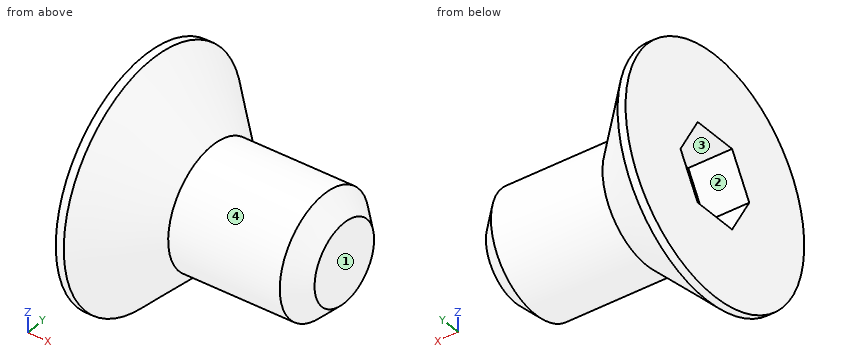
from build123d import *

# Parameters (mm, degrees)
CUT_EXTRUDE1_DEPTH = 1.1


with BuildPart() as part:
    # Sketch1 → Revolve1 (revolve)
    with BuildSketch(Plane.XY, mode=Mode.PRIVATE) as revolve1_sk:
        Polygon((0, -1.5), (2.8, -1.5), (3.3, -1), (3.3, 0), (-1.7, 0), (-1.7, -3), (-1.5, -3), align=None)
    revolve(revolve1_sk.sketch.rotate(Axis((-1.7, 0, 0), (1, 0, 0)), 270), axis=Axis((-1.7, 0, 0), (1, 0, 0)))

    # Sketch2 → Cut-Extrude1 (cut)
    with BuildSketch(Plane.ZY.offset(1.7)):
        Polygon((0, 1.154700538), (-1, 0.577350269), (-1, -0.577350269), (0, -1.154700538), (1, -0.577350269), (1, 0.577350269), align=None)
    extrude(amount=-CUT_EXTRUDE1_DEPTH, mode=Mode.SUBTRACT)


solid = part.part
Work out the finished part from the listing and answer in its coordinate system (mm). Face numbers are marked on the shaded views. Round coordinates to 2 decimals unless told otherwise and drop trailing zeros. Write each loop counter-clockwise with the first axis right and the second up, starting at its lowest first coordinate (ties: lowest second). Pieces come first, ordered by that corner, then holes.
1) The mould has two halves that part along Y. Classify the marked faces 1, 2, 3 and 4: pulls with the +Y half, pulls with the -Y half, needs draft (parallel to the pull), parting line crosses it, or undercut.
2) A cutting plane is placed at B-B (y = 0). Give the vertices of the cut face in (x, z).
3) A cutting plane is placed at A-A (x = -1.25). Give the vertices of the cut face in (y, z).
4) A cutting plane is placed at C-C (x = 0.1). Give the vertices of the cut face in (y, z), plus the area to 3 significant figures.
5) Given pin 1 Ø1.5 at (x, z) = (2.5, -1) entering from +Y; pin 2 Ø1.5 at (x, y) = (1, 1.5) entering from +Z; pin 3 Ø1 at (x, z) = (1, -1.5) entering from -Y, each flat-ended and moving along its own axis, determine where each tip first touches the part or whether it passes through.
6) Straight lines are drawn through the part: line 1 (Z direction, x = 0.45, y = 0.05); line 2 (Y direction, x = -1.4, z = 0.65); line 3 (Y direction, x = -0.9, z = -0.25). For each, find the intervals that lie inside material, in ascending order.
Completed:
1. face 1: needs draft
1. face 2: undercut
1. face 3: undercut
1. face 4: parting line crosses it
2. outline: (-1.7, -3) - (-1.5, -3) - (0, -1.5) - (2.8, -1.5) - (3.3, -1) - (3.3, 1) - (2.8, 1.5) - (0, 1.5) - (-1.5, 3) - (-1.7, 3) - (-1.7, 1) - (-0.6, 1) - (-0.6, -1) - (-1.7, -1) - close
3. outline: circle Ø5.5 at (0, 0); hole (-1.15, 0) - (-0.58, -1) - (0.58, -1) - (1.15, 0) - (0.58, 1) - (-0.58, 1) - close
4. outline: circle Ø3 at (0, 0)
4. area: 7.07 mm2
5. pin 1: stops at y = 1.48
5. pin 2: stops at z = 1.3
5. pin 3: stops at y = -1.12
6. line 1: z = -1.5 to 1.5
6. line 2: y = -2.83 to -0.78, 0.78 to 2.83
6. line 3: y = -2.39 to -1.01, 1.01 to 2.39
